```python
from build123d import *

# Parameters (mm, degrees)
SKETCH1_W              = 127
SKETCH1_H              = 25.4
BOSS_EXTRUDE1_DEPTH    = 6.35
F_10_32_TAPPED_HOLE1_D = 4.0386
F_10_CLEARANCE_HOLE1_D = 5.1054
CHAMFER1_SIZE          = 2.54
CUT_EXTRUDE1_DEPTH     = 7.35


with BuildPart() as part:
    # Sketch1 → Boss-Extrude1 (new body)
    with BuildSketch(Plane(origin=(0, 0, 0), x_dir=(0, 0, -1), z_dir=(1, 0, 0))):
        with Locations((63.5, 12.7)):
            Rectangle(SKETCH1_W, SKETCH1_H)
    extrude(amount=BOSS_EXTRUDE1_DEPTH)

    # #10-32 Tapped Hole1 (through all)
    with Locations(Plane(origin=(6.35, 0, 0), x_dir=(0, 0, -1), z_dir=(1, 0, 0))):
        with Locations((12.7, 12.7), (25.4, 12.7), (38.1, 12.7)):
            Hole(F_10_32_TAPPED_HOLE1_D / 2)

    # #10 Clearance Hole1 (through all)
    with Locations(Plane(origin=(6.35, 0, 0), x_dir=(0, 0, -1), z_dir=(1, 0, 0))):
        with Locations((119.0625, 17.4625), (109.5375, 7.9375)):
            Hole(F_10_CLEARANCE_HOLE1_D / 2)

    # Chamfer1
    chamfer1_edges = [part.edges().sort_by_distance(p)[0] for p in [
        (3.175, 25.4, 0),
        (3.175, 25.4, -127),
        (3.175, 0, -127),
        (3.175, 0, 0),
    ]]
    chamfer(chamfer1_edges, length=CHAMFER1_SIZE)

    # Sketch6 → Cut-Extrude1 (cut, through all)
    with BuildSketch(Plane(origin=(6.35, 0, 0), x_dir=(0, 0, -1), z_dir=(1, 0, 0))):
        with BuildLine():
            Line((93.6625, 7.9375), (58.7375, 7.9375))
            ThreePointArc((58.7375, 7.9375), (53.975, 12.7), (58.7375, 17.4625))
            Line((58.7375, 17.4625), (93.6625, 17.4625))
            ThreePointArc((93.6625, 17.4625), (98.425, 12.7), (93.6625, 7.9375))
        make_face()
    extrude(amount=-CUT_EXTRUDE1_DEPTH, mode=Mode.SUBTRACT)


solid = part.part
```
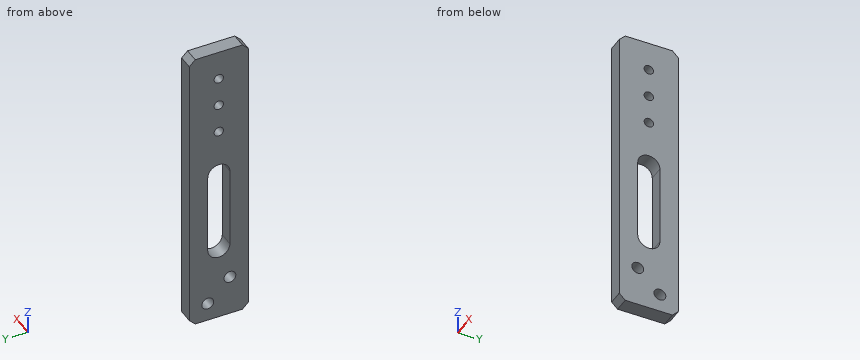
Input: part model. Units: mm. Frame: model coordinates. Give positions to 0.01 mm unless a question says otherwise; leave off trailing zeros. Order: outer loops, then holes, each group sorted by start corner. A loop starts at its lowest first (then second) coordinate and runs counter-clockwise, first axis right, second up. Notation, with made-up numbers: M 42.25,22 L 101.25,22 A31 cw 101.25,60 Z; hole C -20,64.25 d7. An arc over 180 degrees is marked long. One line per question, with ' | ' between items. Start each with the question number.
1. Section query D-D (y = 18.5). Return the cut outline in (x, z).
2. Section query A-A (z = -12.7). Return the cut outline in (x, y), and give its area (3 significant figures).
3. Section query C-C (x = 1.5). Return the cut outline in (y, z) (1 decimal).
4. First-contact query: pin 1 Ø4.5 at (y, z) = (7.94, -109.54) entering from +X. Flat tip, straight axial feed; report the tip coordinate or a pass-through.
5. Section query B-B (y = 12.7). Return the cut outline in (x, z) (3 decimals).
6. Material intervals for probe 1 along Z at (x, y) = (1, 12.75); probe 2 along Y at (x, z) = (1, -63.5); probe 3 along Y at (x, z) = (2.25, -38.1), sorted ascending. Write a range as [from, to].
Here are the results:
1) outline: M 0,-127 L 6.35,-127 L 6.35,-121.39 L 0,-121.39 Z; M 0,-116.73 L 6.35,-116.73 L 6.35,0 L 0,0 Z
2) outline: M 0,0 L 6.35,0 L 6.35,10.68 L 0,10.68 Z; M 0,14.72 L 6.35,14.72 L 6.35,25.4 L 0,25.4 Z | area: 136 mm²
3) outline: M 0,-124.5 L 2.5,-127 L 22.9,-127 L 25.4,-124.5 L 25.4,-2.5 L 22.9,0 L 2.5,0 L 0,-2.5 Z; hole C 7.9,-109.5 d5.1; hole M 7.9,-93.7 A4.8 ccw 17.5,-93.7 L 17.5,-58.7 A4.8 ccw 7.9,-58.7 Z; hole C 12.7,-38.1 d4; hole C 12.7,-25.4 d4; hole C 12.7,-12.7 d4; hole C 17.5,-119.1 d5.1
4) pin 1: through
5) outline: M 0,-127 L 6.35,-127 L 6.35,-98.425 L 0,-98.425 Z; M 0,-53.975 L 6.35,-53.975 L 6.35,-40.119 L 0,-40.119 Z; M 0,-36.081 L 6.35,-36.081 L 6.35,-27.419 L 0,-27.419 Z; M 0,-23.381 L 6.35,-23.381 L 6.35,-14.719 L 0,-14.719 Z; M 0,-10.681 L 6.35,-10.681 L 6.35,0 L 0,0 Z
6) probe 1: [-127, -98.42], [-53.98, -40.12], [-36.08, -27.42], [-23.38, -14.72], [-10.68, 0] | probe 2: [0, 7.94], [17.46, 25.4] | probe 3: [0, 10.68], [14.72, 25.4]
